```python
from build123d import *

# Parameters (mm, degrees)
SKETCH1_W           = 250
SKETCH1_H           = 250
SKETCH1_R           = 4.125
SKETCH1_R_2         = 11.5
SKETCH1_W_2         = 200
SKETCH1_H_2         = 145
BOSS_EXTRUDE1_DEPTH = 3


with BuildPart() as part:
    # Sketch1 → Boss-Extrude1 (new body)
    with BuildSketch(Plane.XY):
        Rectangle(SKETCH1_W, SKETCH1_H)
        with Locations((-115, 115)):
            Circle(SKETCH1_R, mode=Mode.SUBTRACT)
        with Locations((115, 115)):
            Circle(SKETCH1_R, mode=Mode.SUBTRACT)
        with Locations((115, -115)):
            Circle(SKETCH1_R, mode=Mode.SUBTRACT)
        with Locations((-115, -115)):
            Circle(SKETCH1_R, mode=Mode.SUBTRACT)
        with Locations((-77, -85)):
            Circle(SKETCH1_R_2, mode=Mode.SUBTRACT)
        with Locations((0, -85)):
            Circle(SKETCH1_R_2, mode=Mode.SUBTRACT)
        with Locations((77, -85)):
            Circle(SKETCH1_R_2, mode=Mode.SUBTRACT)
        with Locations((0, 22.5)):
            Rectangle(SKETCH1_W_2, SKETCH1_H_2, mode=Mode.SUBTRACT)
    extrude(amount=BOSS_EXTRUDE1_DEPTH)


solid = part.part
```
Could you check a few things on this model? Use its own coordinates, in mm. Give positions to 0.01 mm unless a question says otherwise; leave off trailing zeros. Write each loop counter-clockwise with the first axis right and the second up, starting at its lowest first coordinate (ties: lowest second). Pieces come first, ordered by that corner, then holes. Notation, with made-up numbers: (22, -21) -> (31, -21) arc R26 cw to (31, 14) -> close; hole circle Ø6 at (-27.75, -4.75). An arc over 180 degrees is marked (long way). Write each question's results on one line, items separated by ' | '.
1. Will this pin go through, and if not, where does the flat tip stop? pin 1 Ø13 at (x, y) = (-115, -115) entering from +Z.
Check sheet entries:
pin 1: stops at z = 3
2. I want a section at B-B, the plane x = -115. Write out the boundary of the cut face in (y, z) (3 decimals).
Check sheet entries:
outline: (-125, 0) -> (-119.125, 0) -> (-119.125, 3) -> (-125, 3) -> close; (-110.875, 0) -> (110.875, 0) -> (110.875, 3) -> (-110.875, 3) -> close; (119.125, 0) -> (125, 0) -> (125, 3) -> (119.125, 3) -> close
3. I need wall thicknesses on L1, parallel to Y at x = -115, z = 1.85 (3 decimals); L2, parallel to X at y = -27.5, z = 2; L3, parallel to Y at x = -94, z = 1.5. Which ranges of each line are inside material? Lowest first, please.
Check sheet entries:
L1: y = -125 to -119.125, -110.875 to 110.875, 119.125 to 125 | L2: x = -125 to -100, 100 to 125 | L3: y = -125 to -50, 95 to 125
4. If we mould it in two halves opening along Y, with no side actions, what happens to faces 1 (the flat face through (-2, -54, 0)), 2 (the cylindrical face through (119, 116, 1)), 3 (the cylindrical face through (-111, 116, 1))? For each: released by +Y, released by -Y, zero draft, split by the parting line, or undercut.
Check sheet entries:
face 1: zero draft | face 2: undercut | face 3: undercut
5. I want a section at A-A, the plane y = -10.5. Write out the boundary of the cut face in (x, z), then the cut area to 3 significant figures.
Check sheet entries:
outline: (-125, 0) -> (-100, 0) -> (-100, 3) -> (-125, 3) -> close; (100, 0) -> (125, 0) -> (125, 3) -> (100, 3) -> close | area: 150 mm²
6. I want a section at D-D, the plane x = 27. Write out the boundary of the cut face in (y, z).
Check sheet entries:
outline: (-125, 0) -> (-50, 0) -> (-50, 3) -> (-125, 3) -> close; (95, 0) -> (125, 0) -> (125, 3) -> (95, 3) -> close
